from build123d import *

# Parameters (mm, degrees)
SKETCH1_R           = 35
SKETCH1_R_2         = 11.65
BOSS_EXTRUDE1_DEPTH = 4
CUT_EXTRUDE1_DEPTH  = 10
SKETCH6_R           = 1
CUT_EXTRUDE4_DEPTH  = 10
BOSS_EXTRUDE3_START = 1
SKETCH7_R           = 11.65
SKETCH7_R_2         = 10.65
BOSS_EXTRUDE3_DEPTH = 1
SKETCH8_R           = 11.65
SKETCH8_R_2         = 11.15
CUT_EXTRUDE5_DEPTH  = 0.25
FILLET1_R           = 0.1
CUT_EXTRUDE6_DEPTH  = 1
CUT_EXTRUDE12_DEPTH = 6


with BuildPart() as part:
    # Sketch1 → Boss-Extrude1 (new body)
    with BuildSketch(Plane(origin=(0, 0, 0), x_dir=(0, -0.16775650988153862, -0.9858284604292805), z_dir=(1, 0, 0))):
        with Locations(Location((-28.542888787, 18.957113921, 0), (0, 0, 9.65740334))):
            Circle(SKETCH1_R)
        with Locations(Location((-28.542888787, 18.957113921, 0), (0, 0, 9.65740334))):
            Circle(SKETCH1_R_2, mode=Mode.SUBTRACT)
    extrude(amount=BOSS_EXTRUDE1_DEPTH)

    # Sketch2 → Cut-Extrude1 (cut)
    with BuildSketch(Plane.ZY):
        with BuildLine():
            Line((38.375552951, 38.308271509), (48.999843401, 48.932561958))
            Line((48.999843401, 48.932561958), (51.312030188, 52.930544456))
            Line((51.312030188, 52.930544456), (54.007279042, 51.111570475))
            Line((54.007279042, 51.111570475), (50.414056963, 47.518348396))
            Line((50.414056963, 47.518348396), (39.789766514, 36.894057946))
            ThreePointArc((39.789766514, 36.894057946), (39.100348464, 37.618853459), (38.375552951, 38.308271509))
        make_face()
    extrude(amount=-CUT_EXTRUDE1_DEPTH, mode=Mode.SUBTRACT)

    # Sketch6 → Cut-Extrude4 (cut)
    with BuildSketch(Plane(origin=(4, 0, 0), x_dir=(0, 0, -1), z_dir=(1, 0, 0))):
        with Locations((-24.958212841, -4.023282164)):
            Circle(SKETCH6_R)
        with Locations((2.541787159, 23.476717836)):
            Circle(SKETCH6_R)
        with Locations((-52.458212841, 23.476717836)):
            Circle(SKETCH6_R)
        with Locations((-24.958212841, 50.976717836)):
            Circle(SKETCH6_R)
    extrude(amount=-CUT_EXTRUDE4_DEPTH, mode=Mode.SUBTRACT)

    # Sketch7 → Boss-Extrude3 (add)
    with BuildSketch(Plane.ZY.offset(-4).offset(BOSS_EXTRUDE3_START)):
        with Locations((24.958212841, 23.476717836)):
            Circle(SKETCH7_R)
        with Locations((24.958212841, 23.476717836)):
            Circle(SKETCH7_R_2, mode=Mode.SUBTRACT)
    extrude(amount=-BOSS_EXTRUDE3_DEPTH)

    # Sketch8 → Cut-Extrude5 (cut)
    with BuildSketch(Plane.ZY.offset(-3)):
        with Locations((24.958212841, 23.476717836)):
            Circle(SKETCH8_R)
        with Locations((24.958212841, 23.476717836)):
            Circle(SKETCH8_R_2, mode=Mode.SUBTRACT)
    extrude(amount=-CUT_EXTRUDE5_DEPTH, mode=Mode.SUBTRACT)

    # Fillet1
    fillet1_edges = [part.edges().sort_by_distance(p)[0] for p in [
        (3.25, 23.476717836, 13.808212841),
    ]]
    fillet(fillet1_edges, radius=FILLET1_R)

    # Sketch9 → Cut-Extrude6 (cut)
    with BuildSketch(Plane.ZY):
        Polygon((36.254232608, 38.308271509), (48.989739813, 51.043778714), (52.525273719, 47.508244808), (39.789766514, 34.772737603), (39.082659732, 34.065630822), (35.547125827, 37.601164728), align=None)
        Polygon((48.989739813, 48.922458371), (50.403953376, 47.508244808), (40.402946038, 37.507237471), (38.988732476, 38.921451033), align=None, mode=Mode.SUBTRACT)
    extrude(amount=-CUT_EXTRUDE6_DEPTH, mode=Mode.SUBTRACT)

    # Sketch15 → Cut-Extrude12 (cut)
    with BuildSketch(Plane(origin=(4, 2.265244421, 47.825710378), x_dir=(0, 0, -1), z_dir=(1, 0, 0))):
        Polygon((7.620004071, 34.212873731), (9.865582661, 36.458452321), (9.847893929, 36.476141053), (-10.673980141, 56.998015123), (-12.919044171, 54.752951093), (7.602829899, 34.231077023), align=None)
    extrude(amount=-CUT_EXTRUDE12_DEPTH, mode=Mode.SUBTRACT)


solid = part.part
CAD build for the part. Positions are in the model's coordinates, mm. A direction names the side the tool comes from. Give positions to 0.01 mm unless a question says otherwise; leave off trailing zeros. Loops run counter-clockwise (first coordinate to the right, second up) from the corner with the lowest first, then second, coordinate; pieces in that order, holes last. Notation, with made-up numbers: M -3.5,-30 L 18.5,-30 A27 cw 18.5,-1 Z; hole C -32,-27 d8. An arc over 180 degrees is marked long. One line per question, with ' | ' between items. Start each with the question number.
1. 3-axis set-ups, long thin cutter, end or side, ignore diameter. For faces 4 (the face through (2.521, 43.949, 43.185)), 5 (the face through (0, 24, 10)), 6 (the face through (0.493, 43.852, 41.798)): which of +Z, -Z, +X, -X, +Y, -Y reach the whole face in a straight line?
2. Saw through at C-C on y = 8. Give the cut face in (x, z), plus the area to 3 significant figures.
3. Saw through at A-A on y = 42. Give the cut face in (x, z), plus the area to 3 significant figures.
4. Saw through at B-B on x = 2.1. State how many separate pieces and enclosed holes the cut face has, plus the area to 3 significant figures.
5. Probe L1, parallel to Y at x = 1.8, z = 23.5; L2, parallel to Z at x = 1.15, y = 15; L3, parallel to Z at x = 1.3, y = 40.5. List the from-to ranges inside material, lowest first. Write a range as from..to.
6. Flat gauge pins, fed straight in: pin 1 (2.5 mm diameter, centred on y = 23.48, z = -2.54, fed in from +X); pin 2 (1 mm diameter, centred on x = 1.5, y = 25.5, fed in from -Z); pin 3 (1 mm diameter, centred on x = 2.5, y = 44, fed in from -Z); pin 4 (2 mm diameter, centred on x = 1.5, z = 25.5, fed in from -Y). Where does each tip first touch, or does it go through?
7. Two-plate mould, pull along Z, no slides. Class faces 1 (the face through (3, 19, 35)), 2 (the face through (3.493, 26.676, 35.116)), 3 (the face through (4, 16, 17)): pulls with the +Z half, pulls with the -Z half, needs draft (parallel to the pull), parting line crosses it, or undercut.
8. Saw through at D-D on z = 10. Give the cut face in (x, y), plus the area to 3 significant figures.
Result sheet:
1) face 4: +X, -X | face 5: +Z, -Z, -X, +Y, -Y | face 6: -X
2) outline: M 0,-6.43 L 4,-6.43 L 4,56.35 L 0,56.35 Z | area: 251 mm^2
3) outline: M 0,-4.74 L 4,-4.74 L 4,41.24 L 1,41.24 L 1,39.95 L 0,39.95 Z; M 0,47.02 L 1,47.02 L 1,45.73 L 4,45.73 L 4,54.65 L 0,54.65 Z | area: 217 mm^2
4) separate pieces: 1 | enclosed holes: 5 | area: 3,360 mm^2
5) L1: y = -11.49..11.92, 35.04..58.45 | L2: z = -9..16.97, 32.95..58.92 | L3: z = -5.62..39.74, 44.23..55.54
6) pin 1: stops at x = 4 | pin 2: stops at z = -10.01 | pin 3: stops at z = -3.75 | pin 4: stops at y = -11.52
7) face 1: undercut | face 2: undercut | face 3: needs draft
8) outline: M 0,-8.17 L 4,-8.17 L 4,55.12 L 0,55.12 Z | area: 253 mm^2
